from build123d import *

# Parameters (mm, degrees)
BOSS_EXTRUDE1_DEPTH = 6
SKETCH2_R           = 1.5
CUT_EXTRUDE1_DEPTH  = 108.172757733
CHAMFER1_SIZE       = 6


with BuildPart() as part:
    # Sketch1 → Boss-Extrude1 (new body)
    with BuildSketch(Plane(origin=(0, 0, 0), x_dir=(1, 0, 0), z_dir=(0, 1, 0))):
        Polygon((0, 0), (49.074772881, 85), (0, 85), (-65, 85), (-65, 0), align=None)
    extrude(amount=BOSS_EXTRUDE1_DEPTH)

    # Sketch2 → Cut-Extrude1 (cut, through all)
    with BuildSketch(Plane(origin=(0, 6, 0), x_dir=(1, 0, 0), z_dir=(0, 1, 0))):
        with Locations(Location((-20, 72.5, 0), (0, 0, 270))):
            Circle(SKETCH2_R)
        with Locations(Location((0, 72.5, 0), (0, 0, 270))):
            Circle(SKETCH2_R)
    extrude(amount=-CUT_EXTRUDE1_DEPTH, mode=Mode.SUBTRACT)

    # Chamfer1
    chamfer1_edges = [part.edges().sort_by_distance(p)[0] for p in [
        (24.537386441, 0, -42.5),
    ]]
    chamfer(chamfer1_edges, length=CHAMFER1_SIZE - 0.0001)  # a hair under: the kernel refuses the full size


solid = part.part
The model under review builds one solid part; all positions refer to its coordinate system, in mm. Coordinates: 2 decimals unless noted, no trailing zeros. Order: outer loops, then holes, each group sorted by start corner. A loop starts at its lowest first (then second) coordinate and runs counter-clockwise, first axis right, second up. Notation, with made-up numbers: (64, 8) -> (73, 8) arc R16 cw to (73, 37) -> close; hole circle Ø7 at (-29, 72.5). An arc over 180 degrees is marked (long way). Answer in a Markdown table with one row per item.
(1) The part is to be moulded in two halves that separate along X. For faces 1 (the cylindrical face through (0, 3, -71)), 2 (the cylindrical face through (-20, 3, -71)), 3 (the flat face through (-33, 3, 0)), 4 (the flat face through (-65, 3, -43)), say which applies: +X half, -X half, draft (parallel to the pull), parting line (faces both ways), or undercut.
Answers:
| item | result |
|---|---|
| face 1 | undercut |
| face 2 | undercut |
| face 3 | draft |
| face 4 | -X half |
(2) Wall thickness on line 1 along X through (y, z) = (2.3, -72.5); line 2 along X through (y, z) = (4.6, -73); line 3 along Z through (x, y) = (17.5, 4.35): over which ranges is each line inside the solid? List them lowest first.
Answers:
| item | result |
|---|---|
| line 1 | -65 to -21.5, -18.5 to -1.5, 1.5 to 37.59 |
| line 2 | -65 to -21.41, -18.59 to -1.41, 1.41 to 40.53 |
| line 3 | -85 to -33.61 |
(3) Insertion check: pin 1 (2.5 mm diameter, centred on x = 0, z = -72.5, fed in from +Y); pin 2 (3.5 mm diameter, centred on x = -20, z = -72.5, fed in from +Y); pin 3 (3 mm diameter, centred on y = 1, z = -46.5, fed in from +X). Each pin has a flat end and moves straight along its axis. Give the tip position at first contact, or say it passes through.
Answers:
| item | result |
|---|---|
| pin 1 | through |
| pin 2 | y = 6 |
| pin 3 | x = 23.01 |
(4) Consider section C-C (y = 4.4). Write out the cut boundary in (x, z).
Answers:
| item | result |
|---|---|
| outline | (-65, -85) -> (47.23, -85) -> (-1.85, 0) -> (-65, 0) -> close; hole circle Ø3 at (-20, -72.5); hole circle Ø3 at (0, -72.5) |
(5) Consider section A-A (x = -20). Write out the cut boundary in (y, z), plus the area to 3 significant figures.
Answers:
| item | result |
|---|---|
| outline | (0, -85) -> (6, -85) -> (6, -74) -> (0, -74) -> close; (0, -71) -> (6, -71) -> (6, 0) -> (0, 0) -> close |
| area | 492 mm² |
(6) Consider section B-B (z = -72.5). State how many separate pieces and enclosed holes the cut face has, plus the area to 3 significant figures.
Answers:
| item | result |
|---|---|
| separate pieces | 3 |
| enclosed holes | 0 |
| area | 584 mm² |
